Verification items for the finished model (mm, model axes). Face numbers are marked on the shaded views. Coordinates: 2 decimals unless noted, no trailing zeros. Write each loop counter-clockwise with the first axis right and the second up, starting at its lowest first coordinate (ties: lowest second). Pieces come first, ordered by that corner, then holes. Notation, with made-up numbers: (25.5, 38) -> (53.5, 38) arc R13 cw to (53.5, 48) -> close; hole circle Ø7 at (22.25, 52.25). An arc over 180 degrees is marked (long way). Write item = value, one per line. Start each with the question number.
(1) Material ranges on probe 1 along X at (y, z) = (8.5, 0); probe 2 along Y at (x, z) = (-1.1, 1.6), recorded low to high. Write a range as [from, to].
(2) Gauge pin test, flat end, axial feed: pin 1 Ø1.3 at (x, z) = (-1, 1) entering from +Y. Record the tip position at first contact, or that the pin passes through.
(3) Section check C-C (y = 3.5). Record the cut outline in (x, z).
(4) Mould release check, pull along Y, two halves, no side actions. Record for the marked faces 1, 2 and 3: released by +Y, released by -Y, zero draft, split by the parting line, or undercut.
```python
from build123d import *

# Parameters (mm, degrees)
SKETCH1_R           = 1.75
BOSS_EXTRUDE1_DEPTH = 11.3
SKETCH2_R           = 2.25
BOSS_EXTRUDE2_DEPTH = 0.5
FILLET2_R           = 1


with BuildPart() as part:
    # Sketch1 → Boss-Extrude1 (new, symmetric)
    with BuildSketch(Plane(origin=(0, 0, 0), x_dir=(1, 0, 0), z_dir=(0, 1, 0))):
        with Locations(Location((0, 0, 0), (0, 0, 270))):
            Circle(SKETCH1_R)
    extrude(amount=BOSS_EXTRUDE1_DEPTH, both=True)

    # Sketch2 → Boss-Extrude2 (add, symmetric)
    with BuildSketch(Plane(origin=(0, 11.3, 0), x_dir=(1, 0, 0), z_dir=(0, 1, 0))):
        with Locations(Location((0, 0, 0), (0, 0, 270))):
            Circle(SKETCH2_R)
    boss_extrude2 = extrude(amount=BOSS_EXTRUDE2_DEPTH, both=True)

    # Mirror1: Boss-Extrude2 across plane
    add(boss_extrude2.mirror(Plane.ZX))

    # Fillet2
    fillet2_edges = [part.edges().sort_by_distance(p)[0] for p in [
        (0, -11.8, -2.25),
        (0, 11.8, -2.25),
    ]]
    fillet(fillet2_edges, radius=FILLET2_R - 0.0001)  # a hair under: the kernel refuses the full size


solid = part.part
```
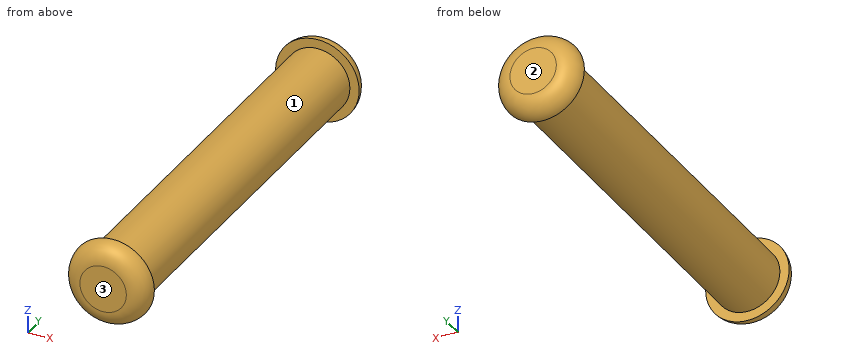
Response:
q1.probe_1 = [-1.75, 1.75]
q1.probe_2 = [-11.52, -10.8], [10.8, 11.52]
q2.pin_1 = 11.8
q3.outline = circle Ø3.5 at (0, 0)
q4.face_1 = undercut
q4.face_2 = released by +Y
q4.face_3 = released by -Y
